Source: CAD feature listing. Evaluate the final solid. Frame: model axes, mm. A direction names the side the tool comes from. Give positions to 0.01 mm unless a question says otherwise; leave off trailing zeros. Loops run counter-clockwise (first coordinate to the right, second up) from the corner with the lowest first, then second, coordinate; pieces in that order, holes last. Notation, with made-up numbers: (88.5, 42) -> (120.5, 42) arc R29 ccw to (120.5, 80) -> close; hole circle Ø7 at (-23, 64). An arc over 180 degrees is marked (long way). Return JSON: item names as keys, results as strings. Group by question number.
(1) Draft query along X for faces 1 (the face through (-2, 1, 0.762)), 2 (the face through (21, 36.809, 13)), 3 (the face through (38.423, 30.964, 12.325)), 4 (the face through (1, -35, 25)). Return one class per face: released by +X, released by -X, zero draft, split by the parting line, or undercut.
(2) Cut plane C-C on y = 0. Return loops of the section in (x, z).
(3) Ray query, line 1 (Y direction, x = -21, z = 23.25); line 2 (Y direction, x = 29, z = 15.25); line 3 (Y direction, x = 15.5, z = 2.25). Return the intervals inside material, ascending. Write a range as from..to.
(4) Cut plane B-B on z = 20. Give the number of separate pieces and of enclosed holes in the cut face, then the cut area to 3 significant figures.
(5) Pin query (flat end, axial travel): pin 1 (7.5 mm diameter, centred on x = 18.5, z = 7, fed in from +Y); pin 2 (8 mm diameter, centred on y = -6.5, z = 19.5, fed in from +X); pin 3 (15 mm diameter, centred on y = 15.5, z = 14, fed in from -X). Return the tip coordinate at first contact, or that it passes through.
(6) Access query for faces 5 (the face through (-22, -7.078, 12)), 6 (the face through (12.74, -2.71, 12.32)), 7 (the face through (-21, 7.593, 13)). Directions: +Z, -Z, +X, -X, +Y, -Y. A direction counts if a zero-diameter tool reaches every point of the face in a straight line with its end or side. Return the directions, or none.
(7) Cut plane A-A on x = 34. Return loops of the section in (y, z).
(8) Cut plane D-D on y = -21.5. Return loops of the section in (x, z).
```python
from build123d import *

# Parameters (mm, degrees)
F2_DEPTH = 25
F3_T     = -0.762
F4_R     = 4.8683707858
F4_R_2   = 4.8302186576
F5_DEPTH = 25


with BuildPart() as f2:
    # F1 (on face) → F2 (new body)
    with BuildSketch(Plane.XY):
        Polygon((0, 9.3792136759), (0, 26.2500010431), (-2.1577780027, 28.9547343873), (-9.2274816707, 37.8164723516), (-35.5537720025, 37.8164723516), (-47.3156645894, 25.2887308598), (-47.3156645894, 11.8099646643), (-26.6031436622, 11.8099646643), (-26.6031436622, 18.618395552), (-18.465153873, 18.618395552), (-18.465153873, 8.3549581468), (-25.3857541829, 8.3549581468), (-25.3857541829, -7.0784804411), (-17.5523422658, -7.0784804411), (-17.5523422658, -17.8431384265), (-27.9656872153, -17.8431384265), (-28.13725546, -12.6960789785), (-47.4213697016, -12.5174866989), (-47.4213697016, -23.0192560703), (-35.9249189496, -36.7836914957), (-9.5176594332, -36.7836914957), (-1.8872555811, -26.7647076398), (0, -17.8735964), align=None)
        Polygon((2.1577780027, 29.1542826942), (0, 26.2500010431), (0, 9.3792136759), (16.634831205, 9.3792136759), (16.634831205, 18.7584273517), (25.1292157918, 18.7584273517), (25.1292157918, 12.0337083936), (0, -17.8735964), (-1.8872555811, -26.7647076398), (-1.8872555811, -35.5147086084), (43.7500029802, -35.5147086084), (43.7500029802, -12.3482472258), (29.1650951026, -12.3482472258), (43.7484294293, 4.4654798699), (43.7484294293, 24.5390101341), (32.9454995436, 37.5711143732), (8.4111846728, 37.5711143732), align=None)
    extrude(amount=F2_DEPTH)

    # F3
    f3_openings = [f2.faces().sort_by_distance(p)[0] for p in [
        (-5.53462, 31.298579, 25),
    ]]
    offset(amount=F3_T, openings=f3_openings, kind=Kind.INTERSECTION)

    # F4 (on face) → F5 (cut)
    with BuildSketch(Plane(origin=(0, 0, 0), x_dir=(1, 0, 0), z_dir=(0, 0, -1))):
        with Locations((-14.3409855664, 0)):
            Circle(F4_R)
        with Locations((27.8169624507, 0)):
            Circle(F4_R_2)
    extrude(amount=-F5_DEPTH, mode=Mode.SUBTRACT)


solid = f2.part
```
Answers:
{
 "1": {"face 1": "undercut", "face 2": "undercut", "face 3": "released by +X", "face 4": "zero draft"},
 "2": {"outline": "(-25.39, 0) -> (-19.21, 0) -> (-19.21, 0.76) -> (-24.62, 0.76) -> (-24.62, 25) -> (-25.39, 25) -> close; (-9.47, 0) -> (0, 0) -> (0, 25) -> (-0.76, 25) -> (-0.76, 0.76) -> (-9.47, 0.76) -> close; (15.02, 0) -> (22.99, 0) -> (22.99, 0.76) -> (16.01, 0.76) -> (16.01, 25) -> (15.02, 25) -> close; (32.65, 0) -> (39.88, 0) -> (39.88, 25) -> (38.87, 25) -> (38.87, 0.76) -> (32.65, 0.76) -> close"},
 "3": {"line 1": "-36.78..-36.02, -18.61..-17.84, -7.08..-6.32, 7.59..8.35, 18.62..19.38, 37.05..37.82", "line 2": "-35.51..-34.75, -13.11..-11.38, 36.81..37.57", "line 3": "-35.51..-34.75, -0.61..0.57, 9.38..10.14, 36.81..37.57"},
 "4": {"separate pieces": "2", "enclosed holes": "2", "area": "428 mm²"},
 "5": {"pin 1": "y = 37.57", "pin 2": "x = 37.71", "pin 3": "x = -47.32"},
 "6": {"face 5": "+Z, -Z, -X", "face 6": "+Z, -Z", "face 7": "+Z"},
 "7": {"outline": "(-35.51, 0) -> (-12.35, 0) -> (-12.35, 25) -> (-13.11, 25) -> (-13.11, 0.76) -> (-34.75, 0.76) -> (-34.75, 25) -> (-35.51, 25) -> close; (-6.77, 0) -> (36.3, 0) -> (36.3, 25) -> (35.11, 25) -> (35.11, 0.76) -> (-5.61, 0.76) -> (-5.61, 25) -> (-6.77, 25) -> close"},
 "8": {"outline": "(-47.42, 0) -> (43.75, 0) -> (43.75, 25) -> (42.99, 25) -> (42.99, 0.76) -> (-46.66, 0.76) -> (-46.66, 25) -> (-47.42, 25) -> close"}
}
